Could you check a few things on this model? Use its own coordinates, in mm. Give positions to 0.01 mm unless a question says otherwise; leave off trailing zeros. Write each loop counter-clockwise with the first axis right and the second up, starting at its lowest first coordinate (ties: lowest second). Pieces come first, ordered by that corner, then holes. Notation, with made-up numbers: (36.5, 83) - (48.5, 83) arc R31 ccw to (48.5, 109) - close; hole circle Ø8 at (56, 48.25). An arc over 180 degrees is marked (long way). Answer as a JSON object with one key per item and string values. Group by question number.
```python
from build123d import *

# Parameters (mm, degrees)
F0_W           = 101.6
F0_H           = 228.6
F1_DEPTH       = 12.7
F3_D           = 4.7625
F3_CSINK_D     = 7.9375
F3_CSINK_ANGLE = 85
F5_D           = 4.7625
F5_CSINK_D     = 7.9375
F5_CSINK_ANGLE = 85


with BuildPart() as f1:
    # F0 (on Top) → F1 (new body)
    with BuildSketch(Plane.XY):
        Rectangle(F0_W, F0_H)
    extrude(amount=F1_DEPTH)

    # F3 (through all)
    with Locations(Plane.XY.offset(12.7)):
        with Locations((-44.45, -107.95), (0, -107.95), (44.45, -107.95)):
            CounterSinkHole(F3_D / 2, F3_CSINK_D / 2, counter_sink_angle=F3_CSINK_ANGLE)

    # F5 (through all)
    with Locations(Plane(origin=(0, 0, 0), x_dir=(1, 0, 0), z_dir=(0, 0, -1))):
        with Locations((44.45, -107.95), (0, -107.95), (-44.45, -107.95)):
            CounterSinkHole(F5_D / 2, F5_CSINK_D / 2, counter_sink_angle=F5_CSINK_ANGLE)


solid = f1.part
```
(1) Will these pins go through, and if not, where does the flat tip stop? P1, Ø8, axis at x = 21, y = 67, coming from the -Z side; P2, Ø7.5, axis at x = 44.45, y = -107.95, coming from the +Z side; P3, Ø6, axis at x = 44.45, y = 107.95, coming from the -Z side.
(2) If we mould it in two halves opening along X, with no side actions, what happens to faces 1 (the flat face through (50.8, -2, 6)), 2 (the flat face through (-1, 114.3, 6)), 3 (the conical face through (2.5, -107.8, 11.1)), 4 (the conical face through (2.5, 107.8, 1.6))? For each: +X half, -X half, draft (parallel to the pull), parting line (faces both ways), or undercut.
(3) I want a section at B-B, the plane x = -44.45. Please give me the cut outline in (y, z), and give its area (3 significant figures).
(4) I want a section at A-A, the plane y = -107.95. Please give me the cut outline in (x, z), and give its area (3 significant figures).
(5) I need wall thicknesses on L1, parallel to Y at x = -44.45, z = 9.75; L2, parallel to X at y = -107.95, z = 4.75. Which ranges of each line are inside material? Lowest first, please.
Entries:
{
 "1": {"P1": "z = 0", "P2": "z = 12.46", "P3": "z = 1.06"},
 "2": {"face 1": "+X half", "face 2": "draft", "face 3": "undercut", "face 4": "undercut"},
 "3": {"outline": "(-114.3, 0) - (-110.33, 0) - (-110.33, 10.97) - (-111.92, 12.7) - (-114.3, 12.7) - close; (-105.57, 0) - (103.98, 0) - (105.57, 1.73) - (105.57, 12.7) - (-103.98, 12.7) - (-105.57, 10.97) - close; (110.33, 1.73) - (111.92, 0) - (114.3, 0) - (114.3, 12.7) - (110.33, 12.7) - close", "area": "2,780 mm^2"},
 "4": {"outline": "(-50.8, 0) - (-46.83, 0) - (-46.83, 10.97) - (-48.42, 12.7) - (-50.8, 12.7) - close; (-42.07, 0) - (-2.38, 0) - (-2.38, 10.97) - (-3.97, 12.7) - (-40.48, 12.7) - (-42.07, 10.97) - close; (2.38, 0) - (42.07, 0) - (42.07, 10.97) - (40.48, 12.7) - (3.97, 12.7) - (2.38, 10.97) - close; (46.83, 0) - (50.8, 0) - (50.8, 12.7) - (48.42, 12.7) - (46.83, 10.97) - close", "area": "1,100 mm^2"},
 "5": {"L1": "-114.3 to -110.33, -105.57 to 105.57, 110.33 to 114.3", "L2": "-50.8 to -46.83, -42.07 to -2.38, 2.38 to 42.07, 46.83 to 50.8"}
}
